Check sheet for the modelled part. Datum: model origin and axes. Units: mm. A direction names the side the tool comes from. Round coordinates to 2 decimals unless told otherwise and drop trailing zeros. Loops run counter-clockwise (first coordinate to the right, second up) from the corner with the lowest first, then second, coordinate; pieces in that order, holes last. Notation, with made-up numbers: (57, 27) - (71, 27) arc R23 cw to (71, 61) - close; hole circle Ø1 at (-1.5, 56). An arc over 180 degrees is marked (long way). Put each result on its own line as item: value. Start each with the question number.
Item 1: Section check B-B, the plane x = 2.75. Record the cut outline in (y, z).
Item 2: Material ranges on line 1 along Y through (x, z) = (4.5, -3.25); line 2 along Y through (x, z) = (4, -7.25); line 3 along Y through (x, z) = (6.25, 7.75), recorded low to high.
Item 3: Gauge pin test, flat ends, axial feed: pin 1 Ø3 at (y, z) = (0, -8.5) entering from +X; pin 2 Ø1.3 at (x, y) = (4, 5.5) entering from +Z; pin 3 Ø4 at (x, y) = (3.5, -8.68) entering from +Z; pin 4 Ø0.8 at (x, y) = (4, 5.5) entering from -Z. Record the tip position at first contact, or that the pin passes through.
Item 4: Tool access check on faces 1 (the cylindrical face through (3.12, -7.49, 4.58)), 2 (the cylindrical face through (3, 0, 5)), 3 (the cylindrical face through (3.923, -5.457, -6.632)), 4 (the flat face through (3, -7, -1)). Record the directions out of +Z, -Z, +X, -X, +Y, -Y that give a thin tool (end or side, any length) a straight path to the whole face; none if there is none.
Item 5: Section check D-D, the plane z = 8.5. Record the cut outline in (x, y).
Item 6: Draft check along Z on faces 5 (the flat face through (5, -9, 1)), 6 (the flat face through (3, -7, -3.6)), 7 (the cylindrical face through (3.15, -10.24, -2.28)). Enter one of: pulls with the +Z half, pulls with the -Z half, needs draft (parallel to the pull), parting line crosses it, or undercut.
Item 7: Section check A-A, the plane z = 3.5. Record the cut outline in (x, y).
Item 8: Section check C-C, the plane y = -1. Record the cut outline in (x, z).
from build123d import *

# Parameters (mm, degrees)
SKETCH1_R                                           = 1
BOSS_EXTRUDE1_DEPTH                                 = 7
SKETCH3_W                                           = 1.25
SKETCH3_H                                           = 11.5
CBORE_FOR_M3_HEX_SOCKET_HEAD_CAP_SCREW1_D           = 3.2
CBORE_FOR_M3_HEX_SOCKET_HEAD_CAP_SCREW1_DEPTH       = 6
CBORE_FOR_M3_HEX_SOCKET_HEAD_CAP_SCREW1_CBORE_D     = 6.5
CBORE_FOR_M3_HEX_SOCKET_HEAD_CAP_SCREW1_CBORE_DEPTH = 3.4
CBORE_FOR_M3_HEX_SOCKET_HEAD_CAP_SCREW1_TIP         = 0.96137699
SKETCH9_R                                           = 3.25
CUT_EXTRUDE1_DEPTH                                  = 22.551334231
TAP_DRILL_FOR_M4_TAP1_OUTLINE_R                     = 1.65
TAP_DRILL_FOR_M4_TAP1_OUTLINE_R_2                   = 1
TAP_DRILL_FOR_M4_TAP1_DEPTH                         = 7


# Read off the part's stored shape, not the designer's step: Tap Drill for M4 Tap1
with BuildPart() as part:
    # Sketch1 → Boss-Extrude1 (new body)
    with BuildSketch(Plane(origin=(0, 0, 0), x_dir=(0, 0, -1), z_dir=(1, 0, 0))):
        with BuildLine():
            ThreePointArc((-1, -4.898979486), (-4.993327693, -0.258221909), (-1.5, 4.769696007))
            Line((-1.5, 4.769696007), (-1.5, 6.4))
            Line((-1.5, 6.4), (1.5, 6.4))
            Line((1.5, 6.4), (1.5, 4.769696007))
            ThreePointArc((1.5, 4.769696007), (4.031128874, 2.958039892), (5, 0))
            ThreePointArc((5, 0), (3.872983346, -3.16227766), (1, -4.898979486))
            Line((1, -4.898979486), (1, -12.459935794))
            ThreePointArc((1, -12.459935794), (9.185586535, -8.477912479), (12.5, 0))
            ThreePointArc((12.5, 0), (-8.477912479, 9.185586535), (-1, -12.459935794))
            Line((-1, -12.459935794), (-1, -4.898979486))
        make_face()
        with Locations((-8.5, 0)):
            Circle(SKETCH1_R, mode=Mode.SUBTRACT)
        with Locations((8.5, 0)):
            Circle(SKETCH1_R, mode=Mode.SUBTRACT)
    extrude(amount=BOSS_EXTRUDE1_DEPTH)

    # Sketch3 → Tap Drill for M3 Tap2 (revolve, cut)
    with BuildSketch(Plane(origin=(3.5, -8.67945764, 1), x_dir=(0, 1, 0), z_dir=(1, 0, 0))):
        with Locations((0.625, 5.75)):
            Rectangle(SKETCH3_W, SKETCH3_H)
    revolve(axis=Axis((3.5, -8.67945764, -5.35), (0, 0, 1)), mode=Mode.SUBTRACT)

    # CBORE for M3 Hex Socket Head Cap Screw1
    with Locations(Plane(origin=(0, 0, -7), x_dir=(-1, 0, 0), z_dir=(0, 0, -1))):
        with Locations((-3.5, -8.67945764)):
            CounterBoreHole(CBORE_FOR_M3_HEX_SOCKET_HEAD_CAP_SCREW1_D / 2, CBORE_FOR_M3_HEX_SOCKET_HEAD_CAP_SCREW1_CBORE_D / 2, CBORE_FOR_M3_HEX_SOCKET_HEAD_CAP_SCREW1_CBORE_DEPTH, depth=CBORE_FOR_M3_HEX_SOCKET_HEAD_CAP_SCREW1_DEPTH)
            with Locations((0, 0, -(CBORE_FOR_M3_HEX_SOCKET_HEAD_CAP_SCREW1_DEPTH + CBORE_FOR_M3_HEX_SOCKET_HEAD_CAP_SCREW1_TIP / 2))):  # 118° drill point
                Cone(0, CBORE_FOR_M3_HEX_SOCKET_HEAD_CAP_SCREW1_D / 2, CBORE_FOR_M3_HEX_SOCKET_HEAD_CAP_SCREW1_TIP, mode=Mode.SUBTRACT)

    # Sketch9 → Cut-Extrude1 (cut, through all)
    with BuildSketch(Plane(origin=(0, 0, -3.6), x_dir=(-1, 0, 0), z_dir=(0, 0, -1))):
        with Locations(Location((-3.5, -8.67945764, 0), (0, 0, 90))):
            Circle(SKETCH9_R)
    extrude(amount=CUT_EXTRUDE1_DEPTH, mode=Mode.SUBTRACT)

    # Tap Drill for M4 Tap1 outline → Tap Drill for M4 Tap1 (cut)
    # profile 1 of 2: a face of its own
    with BuildSketch(Plane.YZ):
        with Locations((0, 8.5)):
            Circle(TAP_DRILL_FOR_M4_TAP1_OUTLINE_R)
        with Locations((0, 8.5)):
            Circle(TAP_DRILL_FOR_M4_TAP1_OUTLINE_R_2, mode=Mode.SUBTRACT)
    # profile 2 of 2: a face of its own
    with BuildSketch(Plane.YZ):
        with Locations((0, -8.5)):
            Circle(TAP_DRILL_FOR_M4_TAP1_OUTLINE_R)
        with Locations((0, -8.5)):
            Circle(TAP_DRILL_FOR_M4_TAP1_OUTLINE_R_2, mode=Mode.SUBTRACT)
    extrude(amount=TAP_DRILL_FOR_M4_TAP1_DEPTH, mode=Mode.SUBTRACT)


solid = part.part
Check result:
1. outline: (-12.46, -1) arc R12.5 ccw to (-11.84, -4) - (-11.84, -3.6) - (-10.09, -3.6) - (-10.09, -1) - close; (-12.46, 1) - (-9.68, 1) - (-9.68, 7.91) arc R12.5 ccw to start; (-7.68, 1) - (-4.9, 1) arc R5 cw to (4.77, 1.5) - (6.4, 1.5) - (6.4, -1.5) - (4.77, -1.5) arc R5 cw to (-4.9, -1) - (-7.27, -1) - (-7.27, -3.6) - (-5.52, -3.6) - (-5.52, -11.22) arc R12.5 ccw (long way) to (-7.68, 9.86) - close; hole circle Ø3.3 at (0, -8.5); hole circle Ø3.3 at (0, 8.5)
2. line 1: -12.07 to -9.93, -7.43 to -3.8, 3.8 to 12.07
2. line 2: -5.47 to -1.08, 1.08 to 10.18
2. line 3: -9.81 to -1.47, 1.47 to 9.81
3. pin 1: through
3. pin 2: z = 11.52
3. pin 3: z = 10.57
3. pin 4: z = -11.41
4. face 1: +Z, -Z
4. face 2: +X, -X
4. face 3: -Z
4. face 4: +X, -X, -Y
5. outline: (0, -9.17) - (2.35, -9.17) arc R1.25 cw (long way) to (4.65, -9.17) - (7, -9.17) - (7, -1.65) - (0, -1.65) - close; (0, 1.65) - (7, 1.65) - (7, 9.17) - (0, 9.17) - close
6. face 5: undercut
6. face 6: pulls with the -Z half
6. face 7: needs draft
7. outline: (0, -12) - (7, -12) - (7, -3.57) - (0, -3.57) - close; (0, 3.57) - (7, 3.57) - (7, 12) - (0, 12) - close; hole circle Ø2.5 at (3.5, -8.68)
8. outline: (0, -12.46) - (7, -12.46) - (7, -9.81) - (0, -9.81) - close; (0, -7.19) - (7, -7.19) - (7, -4.9) - (0, -4.9) - close; (0, 4.9) - (7, 4.9) - (7, 7.19) - (0, 7.19) - close; (0, 9.81) - (7, 9.81) - (7, 12.46) - (0, 12.46) - close
